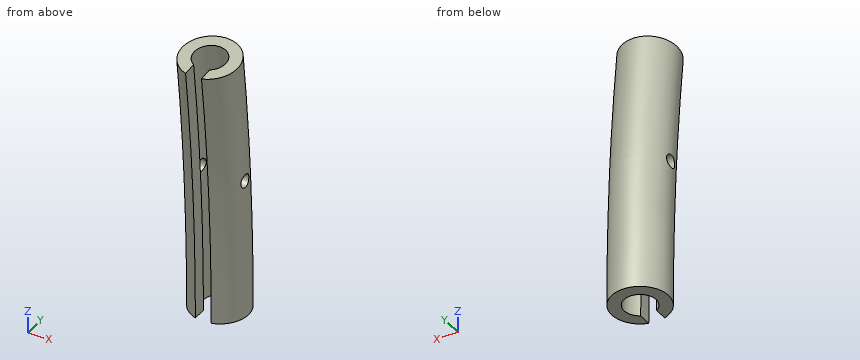
Autodesk Inventor part; units mm, degrees
ref_plane "YZ Plane" through (0, 0, 0) normal (1, 0, 0) x (0, 1, 0)
ref_plane "XZ Plane" through (0, 0, 0) normal (0, 1, 0) x (-1, 0, 0)
ref_plane "XY Plane" through (0, 0, 0) normal (0, 0, 1) x (1, 0, 0)
sketch "Sketch1" plane through (0, 0, 0) normal (1, 0, 0) x (0, 1, 0)
  circle A0 centre (0, 0) radius 1650
  dimension "d0" = 3300
sketch "Sketch2" plane through (0, 0, 0) normal (0, 0, 1) x (1, 0, 0)
  circle A0 centre (0, 1650) radius 21.5
  circle A1 centre (0, 1650) radius 12.2
  line L0 (-30.1, 0) -> (30.1, 0)
  point P0 (0, 0)
  dimension "d1" = 1650
  dimension "d2" = 0
  dimension "d3" = 43
  dimension "d4" = 9.3
revolve "Revolution1" add sketch "Sketch2" angle 7 about axis through (-10, 0, 0) along (1, 0, 0)
sketch "Sketch3" plane through (0, 0, 0) normal (1, 0, 0) x (0, 1, 0)
  line L0 (1642.6517, 530.7226) -> (1398.8963, 530.7226)
  line L1 (1398.8963, 530.7226) -> (1398.8963, -338.3635)
  line L2 (1398.8963, -338.3635) -> (1642.6517, -338.3635)
  line L3 (1642.6517, -338.3635) -> (1642.6517, 530.7226)
  point P0 (0, 0)
extrude "Extrusion1" cut sketch "Sketch3" against normal mid plane 12
sketch "Sketch4" plane through (0, 0, 0) normal (1, 0, 0) x (0, 1, 0)
  circle A0 centre (0, 0) radius 1650
  circle A1 centre (1646.5199, 107.1089) radius 5
  dimension "d8" = 3300
  dimension "d9" = 10
extrude "Extrusion2" cut sketch "Sketch4" along normal mid plane 100 contours A1 A0 | A0 A1 picked at (1644.8813, 106.8012) picked at (1648.186, 107.1089)
equation "\"d0\" = hoop_radius_large"
equation "\"d3\" = od"
equation "\"d4\" = t"
equation "\"d8\" = hoop_radius_large"
equation "\"hoop_radius_large\" = 3300"
equation "\"hoop_width_large\" = 51"
equation "\"hoop_thickness_large\" = 4"
equation "\"hoop_width_medium\" = 33.7"
equation "\"hoop_bushing12_od\" = -2 * hoop_thickness_large + hoop_width_large + hoop_bushing12_radialInterference"
equation "\"hoop_bushing12_radialInterference\" = 0"
equation "\"hoop_angle_z\" = 45deg"
equation "\"hoop_bearing_length\" = 5deg"
equation "\"hoop_cable_diam\" = 5"
equation "\"hoop_cable_pulley_diam\" = 22"
equation "\"hoop_thickness_medium\" = 3.2"
equation "\"hoop_thickness_small\" = 2"
equation "\"hoop_bushing12_thickness\" = -hoop_width_medium + hoop_bushing12_od - 2 * hoop_bushing12_radialInterference"
equation "\"hoop_bushing23_od\" = -2 * hoop_thickness_medium + hoop_width_medium + hoop_bushing23_radialInterference"
equation "\"hoop_bushing23_radialInterference\" = 0"
equation "\"hoop_bushing23_thickness\" = -hoop_width_small + hoop_bushing23_od - 2 * hoop_bushing23_radialInterference"
equation "\"hoop_tabs_hole\" = 12"
equation "\"hoop_tabs_thickness\" = 6"
equation "\"hoop_width_small\" = 25.4"
equation "\"rack_tooth_addendum\" = 5"
equation "\"rack_tooth_dedendum\" = 5"
equation "\"rack_tooth_thickness\" = 5"
equation "\"secure_arm_angle\" = 35deg"
equation "\"secure_arm_radii\" = 9"
equation "\"sm_varx_member_tolerance\" = 0"
equation "\"sm_varx_pinPlate_holeDiameter\" = 5"
equation "\"sm_varx_pinPlate_thickness\" = 5"
equation "\"sm_varx_squareBarThickness\" = 2.5"
equation "\"support_baseClamp_platformLengthBuffer\" = 35"
equation "\"support_baseClamp_platformThickness\" = 15"
equation "\"support_baseClamp_platformWidthBuffer\" = 0"
equation "\"support_baseClamp_sleeveHoleDiameter\" = 12"
equation "\"support_baseClamp_sleeveSweepTerminationAngle\" = 55deg"
equation "\"support_baseClamp_thickness\" = 8"
equation "\"support_frame_endHoleBuffer\" = 45"
equation "\"support_frame_squareBarFillet\" = 2"
equation "\"support_frame_squareBarThickness\" = 5"
equation "\"wheelchair_deployed_height\" = 914"
equation "\"wheelchair_deployed_length\" = 1067"
equation "\"wheelchair_deployed_width\" = 635"
equation "\"od\" = hoop_bushing12_od"
equation "\"t\" = hoop_bushing12_thickness"
equation "\"wheelchatir_pos_deploy_angle_0\" = 65deg"
equation "\"wheelchatir_pos_store_angle_0\" = 90deg"
equation "\"wheelchatir_pos_deploy_angle_1\" = 20deg"
equation "\"wheelchatir_pos_store_angle_1\" = 20deg"
properties part number "large_bearings" material "Polyurethane"
Check sheet for the modelled part. Datum: model origin and axes. Units: mm. Round coordinates to 2 decimals unless told otherwise and drop trailing zeros. Write each loop counter-clockwise with the first axis right and the second up, starting at its lowest first coordinate (ties: lowest second). Pieces come first, ordered by that corner, then holes. Notation, with made-up numbers: M -23,31 L -7,31 A28 cw -7,55 Z; hole C 24.25,-8 d7. An arc over 180 degrees is marked long. Write item = value, one per line. Start each with the question number.
1. Scan lines: line 1 (X direction, y = 1652, z = 118); line 2 (X direction, y = 1649, z = 10); line 3 (Y direction, x = 13, z = 111). Record each from-to range of solid material in increasing order. Write a range as [from, to].
2. Section check A-A, the plane x = -18.5. Record the cut outline in (y, z).
3. Gauge pin test, flat ends, axial feed: pin 1 (1 mm diameter, centred on y = 1659, z = 47, fed in from -X); pin 2 (1.5 mm diameter, centred on x = -10.5, z = 51, fed in from +Y); pin 3 (24.5 mm diameter, centred on y = 1628.5, z = 131, fed in from -X). Record the tip position at first contact, or that the pin passes through.
4. Section check B-B, the plane x = 1. Record the cut outline in (y, z), then the cut area to 3 significant figures.
Results found:
q1.line_1 = [-20.58, -10.5], [10.5, 20.58]
q1.line_2 = [-21.48, -12.16], [12.16, 21.48]
q1.line_3 = [1629.1, 1643.38], [1649.66, 1663.43]
q2.outline = M 1626.83,199.75 A1639.05 cw 1639.05,0 L 1660.95,0 A1660.95 ccw 1648.57,202.42 Z; hole C 1646.52,107.11 d10
q3.pin_1 = -19.45
q3.pin_2 = 1668.38
q3.pin_3 = -21.13
q4.outline = M 1649.77,202.57 A1662.16 cw 1662.16,0 L 1671.48,0 A1671.48 ccw 1659.02,203.7 Z
q4.area = 1,900 mm^2
